```python
from build123d import *

# Parameters (mm, degrees)
F0_R     = 7.576774
F0_W     = 15.357372
F0_H     = 28.439574
F1_DEPTH = 12.7
F2_DEPTH = 50.8
F4_DEPTH = 113.948894
F5_DEPTH = 113.948894


with BuildPart() as f1:
    # F0 (on Top) → F1 (new body)
    with BuildSketch(Plane.XY):
        with BuildLine():
            ThreePointArc((49.864054, -14.219787), (64.083841, 0), (49.864054, 14.219787))
            Line((49.864054, 14.219787), (-34.506682, 14.219787))
            Line((-34.506682, 14.219787), (-34.506682, -14.219787))
            Line((-34.506682, -14.219787), (49.864054, -14.219787))
        make_face()
        with Locations((18.390924, 0)):
            Circle(F0_R, mode=Mode.SUBTRACT)
        with Locations((49.864054, 0)):
            Circle(F0_R, mode=Mode.SUBTRACT)
        with Locations((-42.185368, 0)):
            Rectangle(F0_W, F0_H)
    extrude(amount=F1_DEPTH)

    # F0 (on Top) → F2 (join)
    with BuildSketch(Plane.XY):
        with Locations((-42.185368, 0)):
            Rectangle(F0_W, F0_H)
    extrude(amount=F2_DEPTH)

    # F3 (on face) → F4 (cut, through all)
    with BuildSketch(Plane(origin=(-49.864054, 0, 0), x_dir=(0, -1, 0), z_dir=(-1, 0, 0))):
        with BuildLine():
            ThreePointArc((7.478881, 46.221647), (12.420758, 41.05043), (14.219787, 34.127489))
            Line((14.219787, 34.127489), (14.219787, 50.8))
            Line((14.219787, 50.8), (7.478881, 50.8))
            Line((7.478881, 50.8), (7.478881, 46.221647))
        make_face()
        with BuildLine():
            Line((7.478881, 34.127489), (7.478881, 46.221647))
            Line((7.478881, 46.221647), (7.478881, 50.8))
            Line((7.478881, 50.8), (-7.478881, 50.8))
            Line((-7.478881, 50.8), (-7.478881, 46.221647))
            Line((-7.478881, 46.221647), (-7.478881, 34.127489))
            ThreePointArc((-7.478881, 34.127489), (0, 26.648607), (7.478881, 34.127489))
        make_face()
        with BuildLine():
            Line((-7.478881, 46.221647), (-7.478881, 50.8))
            Line((-7.478881, 50.8), (-14.219787, 50.8))
            Line((-14.219787, 50.8), (-14.219787, 34.127489))
            ThreePointArc((-14.219787, 34.127489), (-12.420758, 41.05043), (-7.478881, 46.221647))
        make_face()
    extrude(amount=-F4_DEPTH, mode=Mode.SUBTRACT)

    # F3 (on face) → F5 (cut, through all)
    with BuildSketch(Plane(origin=(-49.864054, 0, 0), x_dir=(0, -1, 0), z_dir=(-1, 0, 0))):
        with BuildLine():
            ThreePointArc((7.478881, 46.221647), (12.420758, 41.05043), (14.219787, 34.127489))
            Line((14.219787, 34.127489), (14.219787, 50.8))
            Line((14.219787, 50.8), (7.478881, 50.8))
            Line((7.478881, 50.8), (7.478881, 46.221647))
        make_face()
        with BuildLine():
            Line((7.478881, 34.127489), (7.478881, 46.221647))
            Line((7.478881, 46.221647), (7.478881, 50.8))
            Line((7.478881, 50.8), (-7.478881, 50.8))
            Line((-7.478881, 50.8), (-7.478881, 46.221647))
            Line((-7.478881, 46.221647), (-7.478881, 34.127489))
            ThreePointArc((-7.478881, 34.127489), (0, 26.648607), (7.478881, 34.127489))
        make_face()
        with BuildLine():
            Line((-7.478881, 46.221647), (-7.478881, 50.8))
            Line((-7.478881, 50.8), (-14.219787, 50.8))
            Line((-14.219787, 50.8), (-14.219787, 34.127489))
            ThreePointArc((-14.219787, 34.127489), (-12.420758, 41.05043), (-7.478881, 46.221647))
        make_face()
    extrude(amount=-F5_DEPTH, mode=Mode.SUBTRACT)


solid = f1.part
```
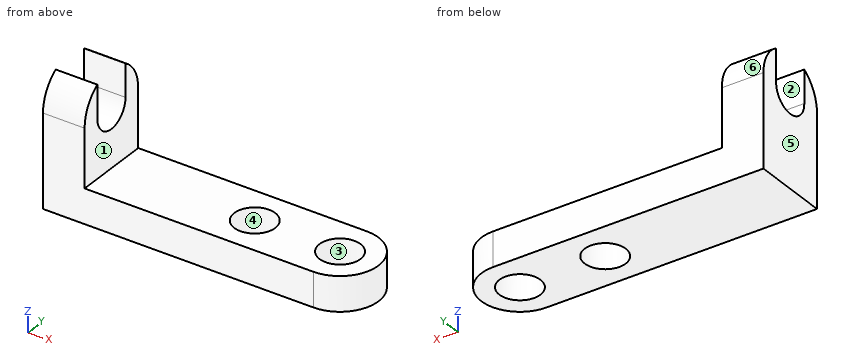
The model under review builds one solid part; all positions refer to its coordinate system, in mm. Face numbers are marked on the shaded views. A direction names the side the tool comes from. Round coordinates to 2 decimals unless told otherwise and drop trailing zeros. Loops run counter-clockwise (first coordinate to the right, second up) from the corner with the lowest first, then second, coordinate; pieces in that order, holes last. Notation, with made-up numbers: M -20,14.25 L 0,14.25 A11 ccw 0,32.25 Z; hole C 79,23 d4. An arc over 180 degrees is marked long. Put each result on its own line as item: value.
Q1. Mouldability with a two-part tool opening along Y and no side actions: class the marked faces 4, 5 and 6 as released by +Y, released by -Y, zero draft, split by the parting line, or undercut.
Result set:
face 4: undercut
face 5: zero draft
face 6: released by +Y
Q2. For pin 1 (6 mm diameter, centred on x = -3.5, y = 11, fed in from -Z); pin 2 (9.5 mm diameter, centred on x = -40.5, z = 43, fed in from +Y); pin 3 (3 mm diameter, centred on y = -10.5, z = 18.5, fed in from +X); pin 4 (4 mm diameter, centred on x = 30, y = -9, fed in from +Z), all flat-tipped, find the tip position at first contact; note any pin that passes through.
Result set:
pin 1: stops at z = 0
pin 2: stops at y = 13.61
pin 3: stops at x = -34.51
pin 4: stops at z = 12.7
Q3. Consider section D-D, the plane z = 5. Give the boundary of the cut face in (x, y).
Result set:
outline: M -49.86,-14.22 L 49.86,-14.22 A14.22 ccw 49.86,14.22 L -49.86,14.22 Z; hole C 18.39,0 d15.15; hole C 49.86,0 d15.15
Q4. Consider section B-B, the plane z = 30. Give the boundary of the cut face in (x, y), then the cut area to 3 significant figures.
Result set:
outline: M -49.86,-14.22 L -34.51,-14.22 L -34.51,-6.24 L -49.86,-6.24 Z; M -49.86,6.24 L -34.51,6.24 L -34.51,14.22 L -49.86,14.22 Z
area: 245 mm²
Q5. To check wall thickness, follow L1, parallel to X at y = 4.25, z = 2; L2, parallel to Z at x = 15, y = 10.25; L3, parallel to X at y = -9, z = 44. State the ranges of each line that lie inside material, in increasing order.
Result set:
L1: x = -49.86 to 12.12, 24.66 to 43.59, 56.14 to 63.43
L2: z = 0 to 12.7
L3: x = -49.86 to -34.51
Q6. Machinability: for the marked faces 1, 2 and 3, which of the approach directions +Z, -Z, +X, -X, +Y, -Y give a long, thin tool a straight path to every point of the face, cutting with its end or side? Answer none if there is none.
Result set:
face 1: +Z, +X, +Y, -Y
face 2: +Z, +X, -X
face 3: +Z, -Z
Q7. Consider section A-A, the plane y = 0. Give the boundary of the cut face in (x, z).
Result set:
outline: M -49.86,0 L 10.81,0 L 10.81,12.7 L -34.51,12.7 L -34.51,26.65 L -49.86,26.65 Z; M 25.97,0 L 42.29,0 L 42.29,12.7 L 25.97,12.7 Z; M 57.44,0 L 64.08,0 L 64.08,12.7 L 57.44,12.7 Z
Q8. Consider section C-C, the plane x = 20. Give the boundary of the cut face in (y, z).
Result set:
outline: M -14.22,0 L -7.4,0 L -7.4,12.7 L -14.22,12.7 Z; M 7.4,0 L 14.22,0 L 14.22,12.7 L 7.4,12.7 Z
